from build123d import *

# Parameters (mm, degrees)
F0_R     = 7.95
F0_R_2   = 3.75
F1_DEPTH = 10
F3_DEPTH = 10
F4_COUNT = 20
F6_DEPTH = 10


with BuildPart() as f1:
    # F0 (on Front) → F1 (new body)
    with BuildSketch(Plane.XZ):
        Circle(F0_R)
        Circle(F0_R_2, mode=Mode.SUBTRACT)
    extrude(amount=F1_DEPTH)

    # F2 (on face) → F3 (join, through all)
    with BuildSketch(Plane.XZ.offset(10)):
        with BuildLine():
            ThreePointArc((-0.831001, 7.906449), (0, 7.95), (0.831001, 7.906449))
            Line((0.831001, 7.906449), (0, 8.95))
            Line((0, 8.95), (-0.831001, 7.906449))
        make_face()
    extrude(amount=-F3_DEPTH)

    # F4: F1 ×20 about axis
    f4_axis = Axis((0, 0, 0), (0, 1, 0))


with BuildPart() as f1_1:
    add(f1.part)
    for i in range(1, F4_COUNT):
        add(f1.part.rotate(f4_axis, i * 360 / F4_COUNT))

    # F5 (on face) → F6 (join, through all)
    with BuildSketch(Plane(origin=(0, 0, 0), x_dir=(-1, 0, 0), z_dir=(0, 1, 0))):
        with BuildLine():
            Line((-0.391982, 3.729457), (0, 3))
            Line((0, 3), (0.391982, 3.729457))
            ThreePointArc((0.391982, 3.729457), (0, 3.75), (-0.391982, 3.729457))
        make_face()
        with BuildLine():
            Line((0, 4.064701), (-0.391982, 3.729457))
            ThreePointArc((-0.391982, 3.729457), (0, 3.75), (0.391982, 3.729457))
            Line((0.391982, 3.729457), (0, 4.064701))
        make_face()
    extrude(amount=-F6_DEPTH)


solid = f1_1.part
Check sheet for the modelled part. Datum: model origin and axes. Units: mm. A direction names the side the tool comes from. Give positions to 0.01 mm unless a question says otherwise; leave off trailing zeros. Write each loop counter-clockwise with the first axis right and the second up, starting at its lowest first coordinate (ties: lowest second). Pieces come first, ordered by that corner, then holes. Notation, with made-up numbers: M 62,-18 L 87,-18 A26 ccw 87,5 Z; hole C -32.75,-13.5 d10. An arc over 180 degrees is marked long. Use one line per item in the form item = value.
(1) Tool access check on faces 1 (the flat face through (-2.22, -5.07, -8.15)), 2 (the flat face through (-4, 0, 0)), 3 (the flat face through (-7.06, -5.07, -4.61)), 4 (the flat face through (-2.2, -5.07, 8.14)), 5 (the flat face through (7.06, -5.07, 4.61)). Record the directions out of +Z, -Z, +X, -X, +Y, -Y that give a thin tool (end or side, any length) a straight path to the whole face; none if there is none.
Answer block:
face_1 = -Z, +Y, -Y
face_2 = +Z, -Z, +X, -X, +Y
face_3 = -X, +Y, -Y
face_4 = +Z, +Y, -Y
face_5 = +X, +Y, -Y
(2) Draft check along Z on faces 6 (the flat face through (7.896, -5.07, 2.996)), 7 (the cylindrical face through (-0.159, -4.93, -3.747)), 8 (the flat face through (0.41, -5.07, -8.436)). Enter one of: pulls with the +Z half, pulls with the -Z half, needs draft (parallel to the pull), parting line crosses it, or undercut.
Answer block:
face_6 = pulls with the +Z half
face_7 = undercut
face_8 = pulls with the -Z half
(3) Material ranges on line 1 along Z through (x, y) = (8.25, -3.25); line 2 along X through (y, z) = (-7.75, 0.5), recorded low to high.
Answer block:
line_1 = -2.86 to -2.37, -0.56 to 0.56, 2.37 to 2.86
line_2 = -8.32 to -3.72, 3.72 to 8.32
(4) Section check B-B on z = 2.5. Record the boundary of the cut face in (x, y), plus the area to 3 significant figures.
Answer block:
outline = M -8.34,-10 L -2.8,-10 L -2.8,0 L -8.34,0 Z; M 2.8,-10 L 8.34,-10 L 8.34,0 L 2.8,0 Z
area = 111 mm2
(5) Section check D-D on x = -4.5. Record the boundary of the cut face in (y, z), plus the area to 3 significant figures.
Answer block:
outline = M -10,-7.03 L 0,-7.03 L 0,7.03 L -10,7.03 Z
area = 141 mm2
(6) Section check C-C on z = 7.5. Record the boundary of the cut face in (x, y), plus the area to 3 significant figures.
Answer block:
outline = M -3.14,-10 L 3.14,-10 L 3.14,0 L -3.14,0 Z
area = 62.9 mm2
(7) Section check A-A on x = 1.25. Record the boundary of the cut face in (y, z).
Answer block:
outline = M -10,-7.85 L 0,-7.85 L 0,-3.54 L -10,-3.54 Z; M -10,3.54 L 0,3.54 L 0,7.85 L -10,7.85 Z
(8) Depth check by flat-ended pin: P1, Ø1, axis at y = -2, z = 2.5, coming from the -X side; P2, Ø1.5, axis at x = -6.5, y = -2.5, coming from the -Z side; P3, Ø1.5, axis at x = -1, y = -4, coming from the +Z side. Enter the tip coordinate at first touch or a pass-through.
Answer block:
P1 = -8.51
P2 = -5.49
P3 = 8.64
